Autodesk Inventor part; units mm, degrees
ref_plane "YZ Plane" through (0, 0, 0) normal (1, 0, 0) x (0, 1, 0)
ref_plane "XZ Plane" through (0, 0, 0) normal (0, 1, 0) x (-1, 0, 0)
ref_plane "XY Plane" through (0, 0, 0) normal (0, 0, 1) x (1, 0, 0)
sketch "Sketch1" plane through (0, 0, 0) normal (0, 1, 0) x (-1, 0, 0)
  circle A0 centre (0, 0) radius 19
  circle A1 centre (0, 0) radius 18
  circle A2 centre (0, 0) radius 15
  dimension "d0" = 38
  dimension "d1" = 36
  dimension "d2" = 30
extrude "Extrusion1" add sketch "Sketch1" along normal blind 29 contours A1
extrude "Extrusion2" add sketch "Sketch1" along normal blind 8.15 contours A0
extrude "Extrusion3" add sketch "Sketch1" along normal blind 29.001 contours A2
extrude "Extrusion4" add sketch "Sketch1" against normal blind 0.001 contours A2
properties part number "NikkonTubelens"
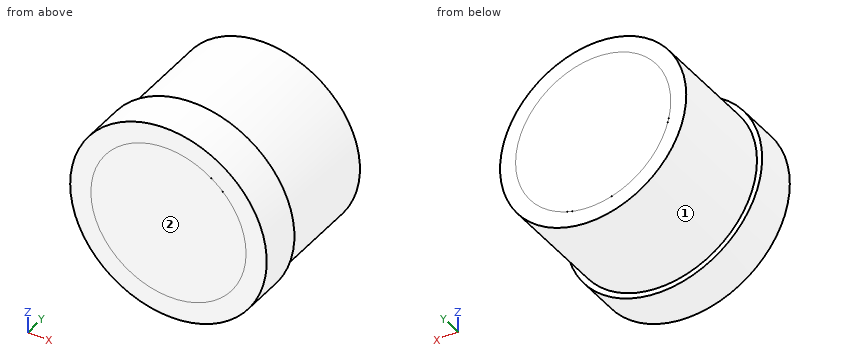
Part model, mm, in its own coordinate system. Face numbers are marked on the shaded views. A direction names the side the tool comes from. Coordinates: 2 decimals unless noted, no trailing zeros. Write each loop counter-clockwise with the first axis right and the second up, starting at its lowest first coordinate (ties: lowest second). Pieces come first, ordered by that corner, then holes.
Item 1: Pin check, flat tips, straight feed: pin 1 (5 mm diameter, centred on y = 17, z = 12, fed in from +X); pin 2 (3 mm diameter, centred on x = 3, y = 25.5, fed in from +Z); pin 3 (6 mm diameter, centred on x = 6, y = 4.5, fed in from -Z). Stop position of each tip, or through.
Item 2: Which spindle directions (+Z, -Z, +X, -X, +Y, -Y) get a long thin tool onto all of the face, cutting with end or side? Do the marked faces 1 and 2. Say none if no direction does.
Item 3: Probe line 1 (Y direction, x = -3, z = -15); line 2 (Y direction, x = 10, z = 15); line 3 (X direction, y = 23, z = -7). List the from-to ranges inside material, lowest first.
Item 4: Slice it at C-C (y = 3.25). Write the cut outline in (x, z).
Item 5: Slice it at D-D (z = 16). Write the cut outline in (x, y), and give its area (3 significant figures).
Results found:
1. pin 1: stops at x = 15.29
1. pin 2: stops at z = 17.94
1. pin 3: stops at z = -18.76
2. face 1: +Y
2. face 2: +Z, -Z, +X, -X, -Y
3. line 1: y = 0 to 29
3. line 2: y = 0 to 8.15
3. line 3: x = -16.58 to 16.58
4. outline: circle Ø38 at (0, 0)
5. outline: (-10.25, 0) - (10.25, 0) - (10.25, 8.15) - (8.25, 8.15) - (8.25, 29) - (-8.25, 29) - (-8.25, 8.15) - (-10.25, 8.15) - close
5. area: 511 mm2
